```python
from build123d import *

# Parameters (mm, degrees)
SKETCH4_W                                           = 70
SKETCH4_H                                           = 77
BOSS_EXTRUDE1_DEPTH                                 = 40
SKETCH5_R                                           = 4
CUT_EXTRUDE1_DEPTH                                  = 30
SKETCH6_W                                           = 30
SKETCH6_H                                           = 30
BOSS_EXTRUDE3_DEPTH                                 = 20
SKETCH7_W                                           = 20
SKETCH7_H                                           = 15
CUT_EXTRUDE2_DEPTH                                  = 30
CSK_FOR_M5_COUNTERSUNK_FLAT_HEAD_SCREW1_D           = 5.5
CSK_FOR_M5_COUNTERSUNK_FLAT_HEAD_SCREW1_DEPTH       = 30
CSK_FOR_M5_COUNTERSUNK_FLAT_HEAD_SCREW1_CSINK_D     = 10.4
CSK_FOR_M5_COUNTERSUNK_FLAT_HEAD_SCREW1_CSINK_ANGLE = 90
CSK_FOR_M5_COUNTERSUNK_FLAT_HEAD_SCREW1_TIP         = 1.652366702
FILLET1_R                                           = 8
FILLET2_R                                           = 2.5


with BuildPart() as part:
    # Sketch4 → Boss-Extrude1 (new body)
    with BuildSketch(Plane(origin=(0, 0, 0), x_dir=(1, 0, 0), z_dir=(0, 1, 0))):
        with Locations((-0.193370166, 0.309392265)):
            Rectangle(SKETCH4_W, SKETCH4_H)
    extrude(amount=BOSS_EXTRUDE1_DEPTH)

    # Sketch5 → Cut-Extrude1 (cut)
    with BuildSketch(Plane(origin=(0, 40, 0), x_dir=(1, 0, 0), z_dir=(0, 1, 0))):
        with Locations(Location((-28.5, 32, 0), (0, 0, 270))):
            Circle(SKETCH5_R)
        with Locations(Location((28.5, 32, 0), (0, 0, 270))):
            Circle(SKETCH5_R)
        with Locations(Location((-28.5, -32, 0), (0, 0, 270))):
            Circle(SKETCH5_R)
        with Locations(Location((28.5, -32, 0), (0, 0, 270))):
            Circle(SKETCH5_R)
    extrude(amount=-CUT_EXTRUDE1_DEPTH, mode=Mode.SUBTRACT)

    # Sketch6 → Boss-Extrude3 (add)
    with BuildSketch(Plane.XY.offset(38.190607735)):
        with Locations((-0.193370166, 20)):
            Rectangle(SKETCH6_W, SKETCH6_H)
    extrude(amount=BOSS_EXTRUDE3_DEPTH)

    # Sketch7 → Cut-Extrude2 (cut)
    with BuildSketch(Plane(origin=(0, 35, 0), x_dir=(1, 0, 0), z_dir=(0, 1, 0))):
        with Locations((-0.193370166, -48.190607735)):
            Rectangle(SKETCH7_W, SKETCH7_H)
    extrude(amount=-CUT_EXTRUDE2_DEPTH, mode=Mode.SUBTRACT)

    # CSK for M5 Countersunk Flat Head Screw1
    with Locations(Plane.XY.offset(58.190607735)):
        with Locations((-0.028758017, 19.958846963)):
            CounterSinkHole(CSK_FOR_M5_COUNTERSUNK_FLAT_HEAD_SCREW1_D / 2, CSK_FOR_M5_COUNTERSUNK_FLAT_HEAD_SCREW1_CSINK_D / 2, depth=CSK_FOR_M5_COUNTERSUNK_FLAT_HEAD_SCREW1_DEPTH, counter_sink_angle=CSK_FOR_M5_COUNTERSUNK_FLAT_HEAD_SCREW1_CSINK_ANGLE)
            with Locations((0, 0, -(CSK_FOR_M5_COUNTERSUNK_FLAT_HEAD_SCREW1_DEPTH + CSK_FOR_M5_COUNTERSUNK_FLAT_HEAD_SCREW1_TIP / 2))):  # 118° drill point
                Cone(0, CSK_FOR_M5_COUNTERSUNK_FLAT_HEAD_SCREW1_D / 2, CSK_FOR_M5_COUNTERSUNK_FLAT_HEAD_SCREW1_TIP, mode=Mode.SUBTRACT)

    # Fillet1
    fillet1_edges = [part.edges().sort_by_distance(p)[0] for p in [
        (34.806629834, 20, 38.190607735),
        (-35.193370166, 20, 38.190607735),
        (-35.193370166, 20, -38.809392265),
        (34.806629834, 20, -38.809392265),
    ]]
    fillet(fillet1_edges, radius=FILLET1_R)

    # Fillet2
    fillet2_edges = [part.edges().sort_by_distance(p)[0] for p in [
        (-15.193370166, 20, 58.190607735),
        (14.806629834, 20, 58.190607735),
    ]]
    fillet(fillet2_edges, radius=FILLET2_R)


solid = part.part
```
Model file for the job. Use its own axes, mm. A direction names the side the tool comes from. Coordinates: 2 decimals unless noted, no trailing zeros. Write each loop counter-clockwise with the first axis right and the second up, starting at its lowest first coordinate (ties: lowest second). Pieces come first, ordered by that corner, then holes. Notation, with made-up numbers: (2, 20) - (18, 20) arc R9 ccw to (18, 36) - close; hole circle Ø4 at (35, -23.5). An arc over 180 degrees is marked (long way). One line per item, written item: value. Start each with the question number.
1. Mould opens along Y. For faces 1 (the conical face through (0.593, 17.158, 55.86)), 2 (the flat face through (0, 24, 40.691)), 3 (the flat face through (-28, 10, -32)) say: released by +Y, released by -Y, zero draft, split by the parting line, or undercut.
2. Flat gauge pins, fed straight in: pin 1 (16.5 mm diameter, centred on y = 24, z = 46.5, fed in from -X); pin 2 (2 mm diameter, centred on x = -20, y = 30, fed in from +Z); pin 3 (10 mm diameter, centred on x = -4, z = 50, fed in from +Y); pin 4 (6.5 mm diameter, centred on x = -28.5, z = 32, fed in from +Y). Where does each tip first touch, or does it go through?
3. Slice it at C-C (x = -28.5). Write the cut outline in (y, z).
4. Tool access for faces 4 (the flat face through (0, 24, 55.691)), 5 (the flat face through (14.807, 20, 47)), 6 (the cylindrical face through (32.466, 25.21, -32.521)): list every direction of +Z, -Z, +X, -X, +Y, -Y with a clear straight run to the whole face (end or side of a thin tool).
5. Slice it at D-D (z = -32). Write the cut outline in (x, y).
6. Probe line 1 (X direction, y = 21, z = -33); line 2 (Z direction, x = 29.5, y = 25.5); line 3 (Z direction, x = -26.5, y = 33). List the from-to ranges inside material, lowest first. Write a range as from..to.
7. Slice it at B-B (z = 32). Write the cut outline in (x, y), plus the area to 3 significant figures.
8. Slice it at A-A (z = 46). Write the cut outline in (x, y), plus the area to 3 significant figures.
Answers below:
1. face 1: undercut
1. face 2: zero draft
1. face 3: released by +Y
2. pin 1: stops at x = -15.19
2. pin 2: stops at z = 38.19
2. pin 3: passes through
2. pin 4: stops at y = 10
3. outline: (0, -38.7) - (40, -38.7) - (40, -36) - (10, -36) - (10, -28) - (40, -28) - (40, 28) - (10, 28) - (10, 36) - (40, 36) - (40, 38.08) - (0, 38.08) - close
4. face 4: +Y, -Y
4. face 5: +Z, +X, +Y, -Y
4. face 6: +Y
5. outline: (-35.1, 0) - (34.72, 0) - (34.72, 40) - (32.5, 40) - (32.5, 10) - (24.5, 10) - (24.5, 40) - (-24.5, 40) - (-24.5, 10) - (-32.5, 10) - (-32.5, 40) - (-35.1, 40) - close
6. line 1: x = -34.89..-32.37, -24.63..24.63, 32.37..34.5
6. line 2: z = -38.34..-35.87, -28.13..28.13, 35.87..37.72
6. line 3: z = -38.81..-35.46, -28.54..28.54, 35.46..38.19
7. outline: (-34.99, 0) - (34.6, 0) - (34.6, 40) - (32.5, 40) - (32.5, 10) - (24.5, 10) - (24.5, 40) - (-24.5, 40) - (-24.5, 10) - (-32.5, 10) - (-32.5, 40) - (-34.99, 40) - close; hole circle Ø5.5 at (-0.03, 19.96)
7. area: 2,280 mm^2
8. outline: (-15.19, 5) - (-10.19, 5) - (-10.19, 35) - (-15.19, 35) - close; (9.81, 5) - (14.81, 5) - (14.81, 35) - (9.81, 35) - close
8. area: 300 mm^2
